Verification items for the finished model (mm, model axes). A direction names the side the tool comes from. Give positions to 0.01 mm unless a question says otherwise; leave off trailing zeros. Write each loop counter-clockwise with the first axis right and the second up, starting at its lowest first coordinate (ties: lowest second). Pieces come first, ordered by that corner, then holes. Notation, with made-up numbers: M 61.25,28.25 L 79.25,28.25 A29 cw 79.25,65.25 Z; hole C 46.5,43 d6. An arc over 180 degrees is marked long. Write item = value, one per line.
from build123d import *

# Parameters (mm, degrees)
CROQUIS1_W              = 20
CROQUIS1_H              = 4
SALIENTE_EXTRUIR1_DEPTH = 3
CROQUIS5_W              = 4
CROQUIS5_H              = 18
CROQUIS5_R              = 1.15
SALIENTE_EXTRUIR2_DEPTH = 3
CROQUIS5_5_R            = 1.15
CORTAR_EXTRUIR3_DEPTH   = 28.073972741
CROQUIS3_R              = 1.05
SALIENTE_EXTRUIR4_DEPTH = 5


with BuildPart() as part:
    # Croquis1 → Saliente-Extruir1 (new body)
    with BuildSketch(Plane.XY):
        with Locations((10, -2)):
            Rectangle(CROQUIS1_W, CROQUIS1_H)
    extrude(amount=SALIENTE_EXTRUIR1_DEPTH)

    # Croquis5 → Saliente-Extruir2 (add)
    # profile 1 of 2: a face of its own
    with BuildSketch(Plane.XY.offset(3)):
        with Locations((2, 9)):
            Rectangle(CROQUIS5_W, CROQUIS5_H)
        with Locations((2, 15.25)):
            Circle(CROQUIS5_R, mode=Mode.SUBTRACT)
    # profile 2 of 2: a face of its own
    with BuildSketch(Plane.XY.offset(3)):
        with Locations((2, 15.25)):
            Circle(CROQUIS5_R)
    extrude(amount=-SALIENTE_EXTRUIR2_DEPTH)

    # Croquis5_5 → Cortar-Extruir3 (cut, through all)
    with BuildSketch(Plane.XY.offset(3)):
        with Locations((2, 15.25)):
            Circle(CROQUIS5_5_R)
    extrude(amount=-CORTAR_EXTRUIR3_DEPTH, mode=Mode.SUBTRACT)

    # Croquis3 → Saliente-Extruir4 (add)
    with BuildSketch(Plane(origin=(0, 0, 0), x_dir=(-1, 0, 0), z_dir=(0, 0, -1))):
        with Locations((-17.5, -2)):
            Circle(CROQUIS3_R)
    extrude(amount=-SALIENTE_EXTRUIR4_DEPTH)


solid = part.part
1) Cross-section at B-B on y = -2. Record the boundary of the cut face in (x, z).
From the geometry:
outline = M 0,0 L 20,0 L 20,3 L 18.55,3 L 18.55,5 L 16.45,5 L 16.45,3 L 0,3 Z
2) Tool access check on faces 1 (the flat face through (20, -2, 1)), 2 (the flat face through (12, 0, 1)). Record the directions out of +Z, -Z, +X, -X, +Y, -Y that give a thin tool (end or side, any length) a straight path to the whole face; none if there is none.
From the geometry:
face_1 = +Z, -Z, +X, +Y, -Y
face_2 = +Z, -Z, +X, +Y
3) Cross-section at A-A on x = 2. Record the boundary of the cut face in (y, z), plus the area to 3 significant figures.
From the geometry:
outline = M -4,0 L 14.1,0 L 14.1,3 L -4,3 Z; M 16.4,0 L 18,0 L 18,3 L 16.4,3 Z
area = 59.1 mm^2
4) Cross-section at D-D on y = 15.25. Record the boundary of the cut face in (x, z).
From the geometry:
outline = M 0,0 L 0.85,0 L 0.85,3 L 0,3 Z; M 3.15,0 L 4,0 L 4,3 L 3.15,3 Z
5) Depth check by flat-ended pin: P1, Ø1.4, axis at x = 2, y = 15.25, coming from the -Z side; P2, Ø0.9, axis at y = 7.5, z = 1.5, coming from the +X side; P3, Ø1, axis at x = 10, z = 2.5, coming from the +Y side. Enter the tip coordinate at first touch or a pass-through.
From the geometry:
P1 = through
P2 = 4
P3 = 0
6) Cross-section at C-C on z = 1.15. Record the boundary of the cut face in (x, y).
From the geometry:
outline = M 0,-4 L 20,-4 L 20,0 L 4,0 L 4,18 L 0,18 Z; hole C 2,15.25 d2.3
7) Draft check along Y on faces 3 (the cylindrical face through (2.53, 14.23, 1.52)), 4 (the flat face through (18, -2, 5)), 5 (the flat face through (2, 18, 2)), 6 (the cylindrical face through (18.33, -2.64, 3.99)). Enter one of: +Y half, -Y half, draft (parallel to the pull), parting line (faces both ways), or undercut.
From the geometry:
face_3 = undercut
face_4 = draft
face_5 = +Y half
face_6 = parting line
8) Material ranges on probe 1 along Y at (x, z) = (2, 1.15); probe 2 along Y at (x, z) = (19, 1.1); probe 3 along X at (y, z) = (3.25, 2.85), recorded low to high. Write a range as from..to.
From the geometry:
probe_1 = -4..14.1, 16.4..18
probe_2 = -4..0
probe_3 = 0..4
